Check sheet for the drawn part. Datum: minimum x, y, z corner. Units: mm. A direction names the side the tool comes from. Round coordinates to 2 decimals unless told otherwise and drop trailing zeros. Loops run counter-clockwise (first coordinate to the right, second up) from the corner with the lowest first, then second, coordinate; pieces in that order, holes last. Notation, with made-up numbers: (74.5, 29) - (80.5, 29) arc R29 ccw to (80.5, 62) - close; hole circle Ø1 at (85.5, 84.25). An arc over 180 degrees is marked (long way). Use CSV: the item, a comma, the result in double quotes.
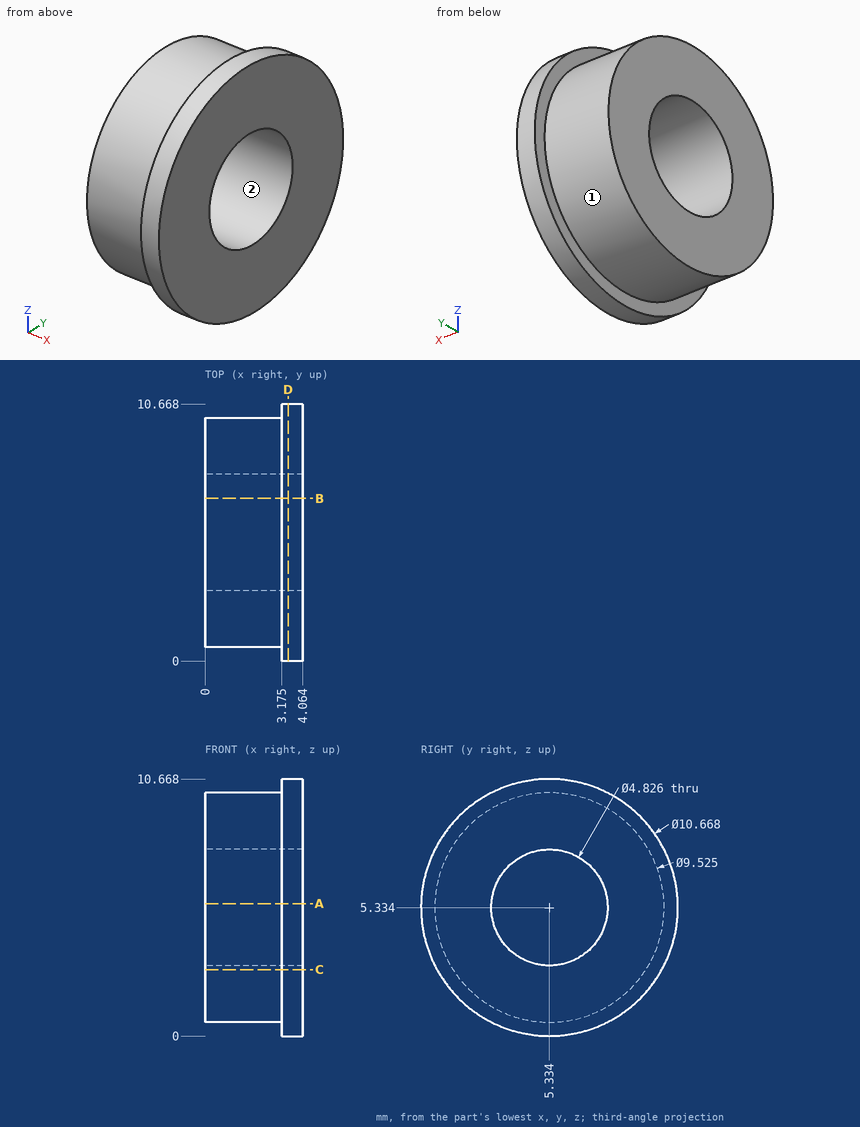
1) Cross-section at C-C, the plane z = 2.75. Record the cut outline in (x, y) (3 decimals).
Returned:
outline,"(0, 1.333) - (3.175, 1.333) - (3.175, 0.668) - (4.064, 0.668) - (4.064, 10) - (3.175, 10) - (3.175, 9.335) - (0, 9.335) - close"
2) Access from +Z, -Z, +X, -X, +Y, -Y to the whole of each face (thin tool, end or side, straight path). Record for the marked faces 1 and 2.
Returned:
face 1,"-X"
face 2,"+X, -X"
3) Gauge pin test, flat ends, axial feed: pin 1 Ø2 at (x, y) = (3, 3.5) entering from +Z; pin 2 Ø5.5 at (y, z) = (5.334, 5.334) entering from -X. Record the tip position at first contact, or that the pin passes through.
Returned:
pin 1,"stops at z = 10.6"
pin 2,"stops at x = 0"
4) Cross-section at D-D, the plane x = 3.45. Record the cut outline in (y, z).
Returned:
outline,"circle Ø10.67 at (5.33, 5.33); hole circle Ø4.83 at (5.33, 5.33)"
5) Cross-section at B-B, the plane y = 6.75. Record the cut outline in (x, z) (3 decimals).
Returned:
outline,"(0, 0.787) - (3.175, 0.787) - (3.175, 0.191) - (4.064, 0.191) - (4.064, 3.38) - (0, 3.38) - close; (0, 7.288) - (4.064, 7.288) - (4.064, 10.477) - (3.175, 10.477) - (3.175, 9.881) - (0, 9.881) - close"
6) Thickness scan on probe 1 along Y at (x, z) = (3.45, 6); probe 2 along Z at (x, y) = (0.5, 7.5); probe 3 along X at (y, z) = (10, 3.25) (3 decimals). Record the ranges inside material, lowest first. Write a range as [from, to].
Returned:
probe 1,"y = [0.04, 3.01], [7.65, 10.63]"
probe 2,"z = [1.09, 4.27], [6.4, 9.58]"
probe 3,"x = [3.175, 4.064]"
7) Cross-section at A-A, the plane z = 5.5. Record the cut outline in (x, y) (3 decimals), then the cut area to 3 significant figures.
Returned:
outline,"(0, 0.574) - (3.175, 0.574) - (3.175, 0.003) - (4.064, 0.003) - (4.064, 2.927) - (0, 2.927) - close; (0, 7.741) - (4.064, 7.741) - (4.064, 10.665) - (3.175, 10.665) - (3.175, 10.094) - (0, 10.094) - close"
area,"20.1 mm²"
